Check sheet for the modelled part. Datum: model origin and axes. Units: mm. A direction names the side the tool comes from. Give positions to 0.01 mm unless a question says otherwise; leave off trailing zeros. Order: outer loops, then holes, each group sorted by start corner. A loop starts at its lowest first (then second) coordinate and runs counter-clockwise, first axis right, second up. Notation, with made-up numbers: M 76.25,-36 L 127.25,-36 A27 cw 127.25,-3 Z; hole C 3.25,72 d2. An arc over 180 degrees is marked long. Return JSON: item names as keys, results as strings. Group by question number.
from build123d import *

# Parameters (mm, degrees)
EXTRUDE_1_DEPTH     = 100
FILLET_1_R          = 4
SKETCH_2_W          = 100
SKETCH_2_H          = 4.232050807
SKETCH_2_H_2        = 4.232050808
EXTRUDE_2_DEPTH     = 24
FILLET_2_R          = 4
FILLET_3_R          = 4
SKETCH_3_R          = 2.1
CUT_EXTRUDE_2_DEPTH = 143.468075254
FILLET_4_R          = 10


with BuildPart() as part:
    # 草图1 → 凸台-拉伸1 (new body)
    with BuildSketch(Plane.XY):
        Polygon((66.282032303, 38.267949192), (0, 0), (0, -20), (94, -20), (94, -26), (-6, -26), (-6, 3.464101615), (63.282032303, 43.464101615), align=None)
    extrude(amount=EXTRUDE_1_DEPTH)

    # 圆角1
    # the kernel refuses this fillet: 4 mm, written as the material it adds along each edge
    with BuildSketch(Plane(origin=(0, 0, 0), x_dir=(0.8660254037844385, 0.5000000000000003, 0), z_dir=(0, 0, 1))) as fillet_1_piece_1:
        with BuildLine():
            CenterArc((FILLET_1_R * 0.57735026919, -FILLET_1_R), FILLET_1_R, 90, 60)
            Line((-FILLET_1_R * 0.288675134595, -FILLET_1_R * 0.5), (0, 0))
            Line((0, 0), (FILLET_1_R * 0.57735026919, 0))
        make_face()
    extrude(amount=100)
    # the kernel refuses this fillet: 4 mm, written as the material it takes off along each edge
    with BuildSketch(Plane(origin=(94, -20, -10), x_dir=(-1, 0, 0), z_dir=(0, 0, 1)), Plane(origin=(94, -26, -10), x_dir=(0, 1, 0), z_dir=(0, 0, 1))) as fillet_1_2_piece_1:
        with BuildLine():
            CenterArc((FILLET_1_R, FILLET_1_R), FILLET_1_R, 180, 90)
            Line((0, FILLET_1_R), (0, 0))
            Line((0, 0), (FILLET_1_R, 0))
        make_face()
    extrude(amount=120, mode=Mode.SUBTRACT)
    with BuildSketch(Plane(origin=(63.282032303, 43.464101615, -10), x_dir=(0.49999999999999706, -0.8660254037844404, 0), z_dir=(0, 0, 1))) as fillet_1_2_piece_2:
        with BuildLine():
            CenterArc((FILLET_1_R, -FILLET_1_R), FILLET_1_R, 90, 90)
            Line((0, -FILLET_1_R), (0, 0))
            Line((0, 0), (FILLET_1_R, 0))
        make_face()
    extrude(amount=120, mode=Mode.SUBTRACT)

    # 草图2 → 凸台-拉伸2 (add)
    with BuildSketch(Plane.ZY.offset(6)):
        with Locations((50, 1.348076212)):
            Rectangle(SKETCH_2_W, SKETCH_2_H)
        with Locations((50, -23.883974596)):
            Rectangle(SKETCH_2_W, SKETCH_2_H_2)
    extrude(amount=EXTRUDE_2_DEPTH)

    # 圆角2
    fillet_2_edges = [part.edges().sort_by_distance(p)[0] for p in [
        (-6, -0.767949192, 50),
        (-6, -21.767949192, 50),
    ]]
    fillet(fillet_2_edges, radius=FILLET_2_R)

    # 圆角3
    fillet_3_edges = [part.edges().sort_by_distance(p)[0] for p in [
        (-6, 3.464101615, 50),
    ]]
    fillet(fillet_3_edges, radius=FILLET_3_R)

    # 草图3 → 切除-拉伸2 (cut, through all)
    with BuildSketch(Plane(origin=(0, 3.464101615, 0), x_dir=(1, 0, 0), z_dir=(0, 1, 0))):
        with Locations(Location((-20, -30, 0), (0, 0, 180))):
            Circle(SKETCH_3_R)
        with Locations(Location((-20, -50, 0), (0, 0, 180))):
            Circle(SKETCH_3_R)
        with Locations(Location((-20, -70, 0), (0, 0, 180))):
            Circle(SKETCH_3_R)
    extrude(amount=-CUT_EXTRUDE_2_DEPTH, mode=Mode.SUBTRACT)

    # 圆角4
    fillet_4_edges = [part.edges().sort_by_distance(p)[0] for p in [
        (0, -20, 50),
    ]]
    fillet(fillet_4_edges, radius=FILLET_4_R)


solid = part.part
1) Depth check by flat-ended pin: P1, Ø8, axis at y = -16.5, z = 53, coming from the +X side; P2, Ø25, axis at x = -13, z = 61, coming from the +Y side; P3, Ø4, axis at y = -8, z = 61, coming from the +X side. Enter the tip coordinate at first touch or a pass-through.
2) Sectioned sample at B-B on z = 70. Record the boundary of the cut face in (x, y), then the cut area to 3 significant figures.
3) Tool access check on faces 1 (the face through (-20.969, -23.854, 48.137)), 2 (the face through (-17.6, -0.768, 49.3)), 3 (the face through (-16, 3.464, 49)), 4 (the face through (34.59, 19.97, 49.3)). Record the directions out of +Z, -Z, +X, -X, +Y, -Y that give a thin tool (end or side, any length) a straight path to the whole face; none if there is none.
4) Sectioned sample at D-D on z = 12.5. Record the boundary of the cut face in (x, y), then the cut area to 3 significant figures.
5) Material ranges on line 1 along Z through (x, y) = (-20, 0.45); line 2 along Y through (x, z) = (30, 85.5); line 3 along Y through (x, z) = (37, 57), recorded low to high.
6) Sectioned sample at A-A on x = -20. State how many separate pieces and enclosed holes the cut face has, then the cut area to 3 significant figures.
7) Release check for a two-part mould opening along Z. For faces 5 (the face through (-20.969, 1.378, 28.137)), 6 (the face through (23, -22, 100)), 7 (the face through (26.92, 22.47, 49.3)) record: released by +Z, released by -Z, zero draft, split by the parting line, or undercut.
8) Sectioned sample at C-C on x = 43.5. Record the boundary of the cut face in (y, z).
Reply:
{
 "1": {"P1": "x = 91.94", "P2": "y = 6.64", "P3": "x = 0"},
 "2": {"outline": "M -30,-26 L -22.1,-26 L -22.1,-21.77 L -30,-21.77 Z; M -30,-0.77 L -22.1,-0.77 L -22.1,3.46 L -30,3.46 Z; M -17.9,-26 L 90,-26 A4 ccw 93.87,-23 A4 ccw 90,-20 L 10,-20 A10 cw 0,-10 L 0,-2.31 A4 cw 2,1.15 L 66.28,38.27 L 65.28,40 A4 ccw 59.82,41.46 L -5.07,4 A4 cw -7.07,3.46 L -17.9,3.46 L -17.9,-0.77 L -10,-0.77 A4 cw -6,-4.77 L -6,-17.77 A4 cw -10,-21.77 L -17.9,-21.77 Z", "area": "1,390 mm^2"},
 "3": {"face 1": "+Y, -Y", "face 2": "+Z, -Z, -X", "face 3": "+Z, -Z, -X, +Y", "face 4": "+Z, -Z, +X"},
 "4": {"outline": "M -30,-26 L 90,-26 A4 ccw 93.87,-23 A4 ccw 90,-20 L 10,-20 A10 cw 0,-10 L 0,-2.31 A4 cw 2,1.15 L 66.28,38.27 L 65.28,40 A4 ccw 59.82,41.46 L -5.07,4 A4 cw -7.07,3.46 L -30,3.46 L -30,-0.77 L -10,-0.77 A4 cw -6,-4.77 L -6,-17.77 A4 cw -10,-21.77 L -30,-21.77 Z", "area": "1,420 mm^2"},
 "5": {"line 1": "0 to 27.9, 32.1 to 47.9, 52.1 to 67.9, 72.1 to 100", "line 2": "-26 to -20, 17.32 to 24.25", "line 3": "-26 to -20, 21.36 to 28.29"},
 "6": {"separate pieces": "8", "enclosed holes": "0", "area": "740 mm^2"},
 "7": {"face 5": "undercut", "face 6": "released by +Z", "face 7": "zero draft"},
 "8": {"outline": "M -26,0 L -20,0 L -20,100 L -26,100 Z; M 25.11,0 L 32.04,0 L 32.04,100 L 25.11,100 Z"}
}
